Source: CAD feature listing. Evaluate the final solid. Frame: model axes, mm. Round coordinates to 2 decimals unless told otherwise and drop trailing zeros. Answer as CSV lines item,"result".
from build123d import *

# Parameters (mm, degrees)
SKETCH1_W               = 635
SKETCH1_H               = 266.7
BOSS_EXTRUDE1_DEPTH     = 6.35
CUT_EXTRUDE2_DEPTH      = 345.425311207
CUT_EXTRUDE2_DEPTH_BACK = 345.425311207
SKETCH2_R               = 4.7625
SKETCH3_R               = 3.96875
CUT_EXTRUDE4_DEPTH      = 345.425311207
SKETCH4_R               = 38.1
CUT_EXTRUDE6_DEPTH      = 345.425311207
SKETCH5_R               = 3.175
CUT_EXTRUDE7_DEPTH      = 345.425311207


with BuildPart() as part:
    # Sketch1 → Boss-Extrude1 (new body)
    with BuildSketch(Plane(origin=(0, 0, 0), x_dir=(1, 0, 0), z_dir=(0, 1, 0))):
        Rectangle(SKETCH1_W, SKETCH1_H)
    extrude(amount=BOSS_EXTRUDE1_DEPTH)

    # Sketch2 → Cut-Extrude2 (cut, two sides: drawn at the far end of the back side and taken through both)
    with BuildSketch(Plane(origin=(0, 0, 0), x_dir=(-1, 0, 0), z_dir=(0, 1, 0)).offset(-CUT_EXTRUDE2_DEPTH_BACK)):
        with Locations(Location((114.3, 0, 0), (0, 0, 90))):
            Circle(SKETCH2_R)
        with Locations(Location((64.3, 0, 0), (0, 0, 90))):
            Circle(SKETCH2_R)
        with Locations(Location((14.3, 0, 0), (0, 0, 90))):
            Circle(SKETCH2_R)
    extrude(amount=CUT_EXTRUDE2_DEPTH + CUT_EXTRUDE2_DEPTH_BACK, mode=Mode.SUBTRACT)

    # Sketch3 → Cut-Extrude4 (cut, through all)
    with BuildSketch(Plane(origin=(0, 0, 0), x_dir=(1, 0, 0), z_dir=(0, 1, 0))):
        with Locations(Location((-292.1, 114.3, 0), (0, 0, 270))):
            Circle(SKETCH3_R)
        with Locations(Location((-292.1, 76.2, 0), (0, 0, 270))):
            Circle(SKETCH3_R)
        with Locations(Location((-292.1, -76.2, 0), (0, 0, 270))):
            Circle(SKETCH3_R)
        with Locations(Location((-292.1, -114.3, 0), (0, 0, 270))):
            Circle(SKETCH3_R)
        with Locations(Location((114.3, 114.3, 0), (0, 0, 270))):
            Circle(SKETCH3_R)
        with Locations(Location((114.3, 76.2, 0), (0, 0, 270))):
            Circle(SKETCH3_R)
        with Locations(Location((114.3, -76.2, 0), (0, 0, 270))):
            Circle(SKETCH3_R)
        with Locations(Location((114.3, -114.3, 0), (0, 0, 270))):
            Circle(SKETCH3_R)
    extrude(amount=CUT_EXTRUDE4_DEPTH, mode=Mode.SUBTRACT)

    # Sketch4 → Cut-Extrude6 (cut, through all)
    with BuildSketch(Plane(origin=(0, 0, 0), x_dir=(1, 0, 0), z_dir=(0, 1, 0))):
        with Locations((317.5, 0)):
            Circle(SKETCH4_R)
    extrude(amount=CUT_EXTRUDE6_DEPTH, mode=Mode.SUBTRACT)

    # Sketch5 → Cut-Extrude7 (cut, through all)
    with BuildSketch(Plane(origin=(0, 6.35, 0), x_dir=(1, 0, 0), z_dir=(0, 1, 0))):
        with Locations(Location((139.7, 114.3, 0), (0, 0, 270))):
            Circle(SKETCH5_R)
        with Locations(Location((165.1, 114.3, 0), (0, 0, 270))):
            Circle(SKETCH5_R)
        with Locations(Location((190.5, 114.3, 0), (0, 0, 270))):
            Circle(SKETCH5_R)
        with Locations(Location((215.9, 114.3, 0), (0, 0, 270))):
            Circle(SKETCH5_R)
        with Locations(Location((241.3, 114.3, 0), (0, 0, 270))):
            Circle(SKETCH5_R)
        with Locations(Location((266.7, 114.3, 0), (0, 0, 270))):
            Circle(SKETCH5_R)
        with Locations(Location((292.1, 114.3, 0), (0, 0, 270))):
            Circle(SKETCH5_R)
        with Locations(Location((165.1, 88.9, 0), (0, 0, 270))):
            Circle(SKETCH5_R)
        with Locations(Location((190.5, 88.9, 0), (0, 0, 270))):
            Circle(SKETCH5_R)
        with Locations(Location((215.9, 88.9, 0), (0, 0, 270))):
            Circle(SKETCH5_R)
        with Locations(Location((241.3, 88.9, 0), (0, 0, 270))):
            Circle(SKETCH5_R)
        with Locations(Location((266.7, 88.9, 0), (0, 0, 270))):
            Circle(SKETCH5_R)
        with Locations(Location((292.1, 88.9, 0), (0, 0, 270))):
            Circle(SKETCH5_R)
        with Locations(Location((165.1, 63.5, 0), (0, 0, 270))):
            Circle(SKETCH5_R)
        with Locations(Location((190.5, 63.5, 0), (0, 0, 270))):
            Circle(SKETCH5_R)
        with Locations(Location((215.9, 63.5, 0), (0, 0, 270))):
            Circle(SKETCH5_R)
        with Locations(Location((241.3, 63.5, 0), (0, 0, 270))):
            Circle(SKETCH5_R)
        with Locations(Location((266.7, 63.5, 0), (0, 0, 270))):
            Circle(SKETCH5_R)
        with Locations(Location((292.1, 63.5, 0), (0, 0, 270))):
            Circle(SKETCH5_R)
        with Locations(Location((139.7, 88.9, 0), (0, 0, 270))):
            Circle(SKETCH5_R)
        with Locations(Location((139.7, 63.5, 0), (0, 0, 270))):
            Circle(SKETCH5_R)
    extrude(amount=-CUT_EXTRUDE7_DEPTH, mode=Mode.SUBTRACT)


solid = part.part
1. Pin query (flat end, axial travel): pin 1 (5.5 mm diameter, centred on x = 292.1, z = -63.5, fed in from -Y). Return the tip coordinate at first contact, or that it passes through.
Results below:
pin 1,"through"
2. Line query: L1, parallel to Z at x = 139.7, y = 3.5 (3 decimals); L2, parallel to X at y = 1.5, z = 0; L3, parallel to X at y = 2.25, z = 76.2. Output: solid intervals per line, ascending. Write a range as [from, to].
Results below:
L1,"[-133.35, -117.475], [-111.125, -92.075], [-85.725, -66.675], [-60.325, 133.35]"
L2,"[-317.5, -119.06], [-109.54, -69.06], [-59.54, -19.06], [-9.54, 279.4]"
L3,"[-317.5, -296.07], [-288.13, 110.33], [118.27, 317.5]"
3. Section query A-A on y = 2.75. Give the number of separate pieces and of enclosed holes in the cut face, and give its area (3 significant figures).
Results below:
separate pieces,"1"
enclosed holes,"32"
area,"166,000 mm2"
